from build123d import *

# Parameters (mm, degrees)
SKETCH_1_R                       = 32.5
SKETCH_1_R_2                     = 20
EXTRUDE_1_DEPTH                  = 2
SKETCH_2_R                       = 8
EXTRUDE_2_DEPTH                  = 2
SKETCH_3_R                       = 3.5
CUT_EXTRUDE_1_DEPTH              = 2
FILLET_1_R                       = 5
PATTERN_CIRCULAR_1_COUNT         = 4
FILLET_1_OF_PATTERN_CIRCULAR_1_R = 5


with BuildPart() as part:
    # 草图1 → 凸台-拉伸1 (new body)
    with BuildSketch(Plane.XY):
        Circle(SKETCH_1_R)
        Circle(SKETCH_1_R_2, mode=Mode.SUBTRACT)
    extrude(amount=EXTRUDE_1_DEPTH)

    # 草图2 → 凸台-拉伸2 (add)
    with BuildSketch(Plane.XY.offset(2)):
        with Locations((24.04163056, 24.04163056)):
            Circle(SKETCH_2_R)
    extrude_2 = extrude(amount=-EXTRUDE_2_DEPTH)

    # 草图3 → 切除-拉伸1 (cut)
    with BuildSketch(Plane.XY.offset(2)):
        with Locations((24.04163056, 24.04163056)):
            Circle(SKETCH_3_R)
    cut_extrude_1 = extrude(amount=-CUT_EXTRUDE_1_DEPTH, mode=Mode.SUBTRACT)

    # 圆角1
    fillet_1_edges = [part.edges().sort_by_distance(p)[0] for p in [
        (16.944361965, 27.733348113, 1),
        (27.733348113, 16.944361965, 1),
    ]]
    fillet(fillet_1_edges, radius=FILLET_1_R)

    # 阵列(圆周)1: 凸台-拉伸2, 切除-拉伸1 ×4 about axis
    pattern_circular_1_axis = Axis((0, 0, 0), (0, 0, 1))
    add([extrude_2.rotate(pattern_circular_1_axis, i * 360 / PATTERN_CIRCULAR_1_COUNT) for i in range(1, PATTERN_CIRCULAR_1_COUNT)])
    add([cut_extrude_1.rotate(pattern_circular_1_axis, i * 360 / PATTERN_CIRCULAR_1_COUNT) for i in range(1, PATTERN_CIRCULAR_1_COUNT)], mode=Mode.SUBTRACT)

    # 圆角1 of 阵列(圆周)1
    fillet_1_of_pattern_circular_1_edges = [part.edges().sort_by_distance(p)[0] for p in [
        (-27.733348113, 16.944361965, 1),
        (-16.944361965, 27.733348113, 1),
        (-16.944361965, -27.733348113, 1),
        (-27.733348113, -16.944361965, 1),
        (27.733348113, -16.944361965, 1),
        (16.944361965, -27.733348113, 1),
    ]]
    fillet(fillet_1_of_pattern_circular_1_edges, radius=FILLET_1_OF_PATTERN_CIRCULAR_1_R)


solid = part.part
CAD build for the part. Positions are in the model's coordinates, mm. Coordinates: 2 decimals unless noted, no trailing zeros. Write each loop counter-clockwise with the first axis right and the second up, starting at its lowest first coordinate (ties: lowest second). Pieces come first, ordered by that corner, then holes. Notation, with made-up numbers: (-13, 53.25) - (12, 53.25) arc R25 ccw to (12, 68.25) - close; hole circle Ø9 at (63.25, 53.5). An arc over 180 degrees is marked (long way). Use a Markdown table: item, result. Add a question column.
Item 1: Band-saw the part on A-A, the plane x = 0. Give the cut face in (y, z), and give its area (3 significant figures).
Item 2: Flat gauge pin, fed straight in: pin 1 (1 mm diameter, centred on x = 16, z = 1, fed in from +Y). Where does the tip first touch, or does it go through?
Item 3: Band-saw the part on D-D, the plane y = -22.5. Give the cut face in (x, z).
Item 4: Band-saw the part on C-C, the plane x = 25.5. Give the cut face in (y, z).
Item 5: Mould opens along X. For faces 1 (the face through (-29.58, 29.814, 1.014)), 2 (the face through (14, -15, 0)), 3 (the face through (-32.5, 0.2, 1)) say: pulls with the +X half, pulls with the -X half, needs draft (parallel to the pull), parting line crosses it, or undercut.
Item 6: Drill centre lines: L1, parallel to Y at x = 24, z = 1.4; L2, parallel to Y at x = 0, z = 1.15. Where is each one in solid material? Low to high. Write a range as from..to.
Numbers:
| question | item | result |
|---|---|---|
| 1 | outline | (-32.5, 0) - (-20, 0) - (-20, 2) - (-32.5, 2) - close; (20, 0) - (32.5, 0) - (32.5, 2) - (20, 2) - close |
| 1 | area | 50.0 mm2 |
| 2 | pin 1 | y = 29.1 |
| 3 | outline | (-31.89, 0) - (-27.18, 0) - (-27.18, 2) - (-31.89, 2) - close; (-20.9, 0) - (20.9, 0) - (20.9, 2) - (-20.9, 2) - close; (27.18, 0) - (31.89, 0) - (31.89, 2) - (27.18, 2) - close |
| 4 | outline | (-31.91, 0) - (-27.22, 0) - (-27.22, 2) - (-31.91, 2) - close; (-20.86, 0) - (20.86, 0) - (20.86, 2) - (-20.86, 2) - close; (27.22, 0) - (31.91, 0) - (31.91, 2) - (27.22, 2) - close |
| 5 | face 1 | undercut |
| 5 | face 2 | needs draft |
| 5 | face 3 | pulls with the -X half |
| 6 | L1 | -32.04..-27.54, -20.54..20.54, 27.54..32.04 |
| 6 | L2 | -32.5..-20, 20..32.5 |
